```python
from build123d import *

# Parameters (mm, degrees)
F1_DEPTH = 53.594


with BuildPart() as f1:
    # F0 (on Front) → F1 (new body)
    with BuildSketch(Plane.XZ):
        with BuildLine():
            Line((-19.50657, -7.33976), (-45.16267, -7.33976))
            Line((-45.16267, -7.33976), (-45.16267, -30.615397))
            Line((-45.16267, -30.615397), (46.485152, -30.615397))
            Line((46.485152, -30.615397), (46.485152, -7.33976))
            Line((46.485152, -7.33976), (19.50657, -7.33976))
            ThreePointArc((19.50657, -7.33976), (0, -20.841746), (-19.50657, -7.33976))
        make_face()
        with BuildLine():
            Line((46.485152, 33.524852), (-45.16267, 33.524852))
            Line((-45.16267, 33.524852), (-45.16267, 8.529992))
            Line((-45.16267, 8.529992), (-19.016246, 8.529992))
            ThreePointArc((-19.016246, 8.529992), (0, 20.841746), (19.016246, 8.529992))
            Line((19.016246, 8.529992), (46.485152, 8.529992))
            Line((46.485152, 8.529992), (46.485152, 33.524852))
        make_face()
        with BuildLine():
            ThreePointArc((19.016246, 8.529992), (0, 20.841746), (-19.016246, 8.529992))
            ThreePointArc((-19.016246, 8.529992), (-20.831805, 0.643636), (-19.50657, -7.33976))
            ThreePointArc((-19.50657, -7.33976), (0, -20.841746), (19.50657, -7.33976))
            ThreePointArc((19.50657, -7.33976), (20.505235, -3.730106), (20.841746, 0))
            ThreePointArc((20.841746, 0), (20.380261, 4.361571), (19.016246, 8.529992))
        make_face()
    extrude(amount=F1_DEPTH)


solid = f1.part
```
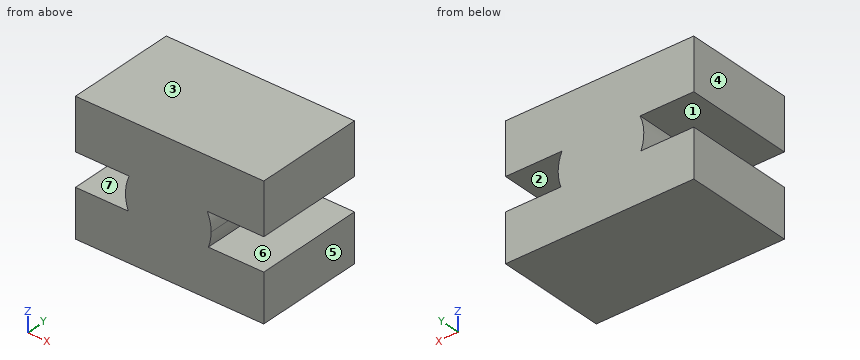
Can you work these out from the model? Positions are in its coordinate system, mm. Face numbers are marked on the shaded views. A direction names the side the tool comes from. Give positions to 0.01 mm unless a question says otherwise; leave off trailing zeros. Loops run counter-clockwise (first coordinate to the right, second up) from the corner with the lowest first, then second, coordinate; pieces in that order, holes last. Notation, with made-up numbers: M 57.5,77.25 L 72.5,77.25 A29 cw 72.5,112.25 Z; hole C 70,64 d11. An arc over 180 degrees is marked long. Answer in a Markdown table with one row per item.
1. Suppose I cut it at C-C on z = -1.5. Write out the boundary of the cut face in (x, y).
Taken from the geometry:
| item | result |
|---|---|
| outline | M -20.79,-53.59 L 20.79,-53.59 L 20.79,0 L -20.79,0 Z |
2. For pin 1 Ø6 at (x, z) = (-33.5, 9.5) entering from +Y; pin 2 Ø12 at (y, z) = (-32.5, 0.5) entering from -X, each with a flat end and sliding along its axis, tell me the tip position at first contact or that it passes through.
Taken from the geometry:
| item | result |
|---|---|
| pin 1 | stops at y = 0 |
| pin 2 | stops at x = -20.84 |
3. Suppose I cut it at A-A on x = -33. Write out the boundary of the cut face in (y, z).
Taken from the geometry:
| item | result |
|---|---|
| outline | M -53.59,-30.62 L 0,-30.62 L 0,-7.34 L -53.59,-7.34 Z; M -53.59,8.53 L 0,8.53 L 0,33.52 L -53.59,33.52 Z |
4. Thinking about a two-plate mould opening in Z: for the marked faces 1, 2, 3 and 4, which applies, released by +Z, released by -Z, zero draft, split by the parting line, or undercut?
Taken from the geometry:
| item | result |
|---|---|
| face 1 | undercut |
| face 2 | undercut |
| face 3 | released by +Z |
| face 4 | zero draft |
5. Suppose I cut it at B-B on y = -26.5. Write out the boundary of the cut face in (x, z), plus the area to 3 significant figures.
Taken from the geometry:
| item | result |
|---|---|
| outline | M -45.16,-30.62 L 46.49,-30.62 L 46.49,-7.34 L 19.51,-7.34 A20.84 ccw 20.84,0 A20.84 ccw 19.02,8.53 L 46.49,8.53 L 46.49,33.52 L -45.16,33.52 L -45.16,8.53 L -19.02,8.53 A20.84 ccw -19.51,-7.34 L -45.16,-7.34 Z |
| area | 5,070 mm² |
6. If I drill on line 1 along Z through (x, y) = (41.5, -33.5); line 2 along X through (y, z) = (-49, 4); line 3 along X through (y, z) = (-43.5, 2.5), over which ranges is the centre line in solid material (lowest first)?
Taken from the geometry:
| item | result |
|---|---|
| line 1 | z = -30.62 to -7.34, 8.53 to 33.52 |
| line 2 | x = -20.45 to 20.45 |
| line 3 | x = -20.69 to 20.69 |
7. Which directions (+Z, -Z, +X, -X, +Y, -Y) give clear straight access to the entire face, cutting with the end or side of a thin tool? Please do the marked faces 5, 6 and 7.
Taken from the geometry:
| item | result |
|---|---|
| face 5 | +Z, -Z, +X, +Y, -Y |
| face 6 | +X, +Y, -Y |
| face 7 | -X, +Y, -Y |
